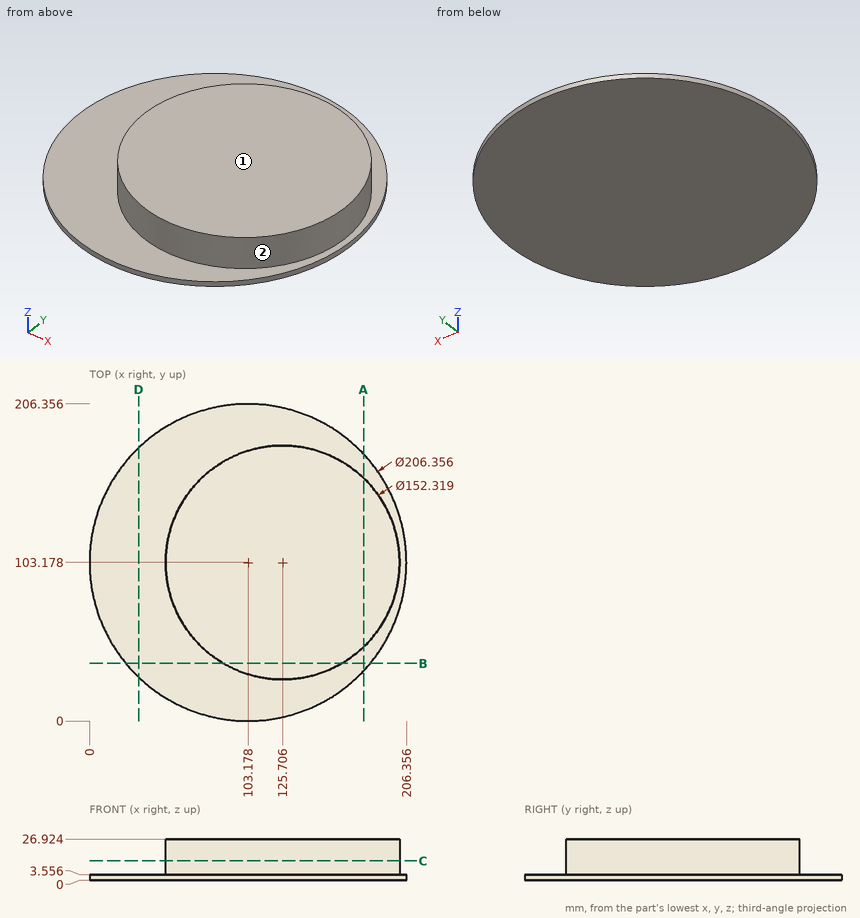
The drawing under review shows one solid part. Ordinate dimensions are in mm from its lowest x, y, z. A direction names the side the tool comes from. Give positions to 0.01 mm unless a question says otherwise; leave off trailing zeros. Loops run counter-clockwise (first coordinate to the right, second up) from the corner with the lowest first, then second, coordinate; pieces in that order, holes last. Notation, with made-up numbers: M -15.75,-13 L 43.25,-13 A21 cw 43.25,18 Z; hole C 32,87.5 d1. An arc over 180 degrees is marked long. Return JSON: item names as keys, results as strings. Group by question number.
Item 1: Tool access review of the marked faces 1 and 2: name each direction out of +Z, -Z, +X, -X, +Y, -Y from which nothing blocks a thin tool from reaching the whole face with its end or side.
Item 2: We need section C-C (z = 12.75). Give the boundary of the cut face in (x, y), and give its area (3 significant figures).
Item 3: For probe 1 along Z at (x, y) = (128, 22); probe 2 along X at (y, z) = (153.5, 7.25) (1 decimal); probe 3 along Y at (x, z) = (37, 3.5) (1 decimal), list the stretches that pass through material, from the lowest coordinate up.
Item 4: We need section D-D (x = 32). Give the boundary of the cut face in (y, z).
Item 5: We need section A-A (x = 178.5). Give the boundary of the cut face in (y, z) (1 decimal), and give its area (3 significant figures).
Item 6: We need section B-B (y = 37.5). Give the boundary of the cut face in (x, z) (1 decimal), and give its area (3 significant figures).
Item 7: Insertion check: pin 1 Ø2 at (y, z) = (95.5, 6) entering from -X; pin 2 Ø8 at (y, z) = (42.5, 20) entering from -X (1 decimal); pin 3 Ø5 at (x, z) = (167.5, 24) entering from -Y. Each pin has a flat end and moves straight along its axis. Give the tip position at first contact, or say it passes through.
Output:
{
 "1": {"face 1": "+Z, +X, -X, +Y, -Y", "face 2": "+Z"},
 "2": {"outline": "C 125.71,103.18 d152.32", "area": "18,200 mm^2"},
 "3": {"probe 1": "z = 0 to 3.56", "probe 2": "x = 68.5 to 182.9", "probe 3": "y = 24 to 182.3"},
 "4": {"outline": "M 28.48,0 L 177.87,0 L 177.87,3.56 L 28.48,3.56 Z"},
 "5": {"outline": "M 32.7,0 L 173.7,0 L 173.7,3.6 L 158.1,3.6 L 158.1,26.9 L 48.3,26.9 L 48.3,3.6 L 32.7,3.6 Z", "area": "3,070 mm^2"},
 "6": {"outline": "M 23.6,0 L 182.8,0 L 182.8,3.6 L 164.3,3.6 L 164.3,26.9 L 87.1,26.9 L 87.1,3.6 L 23.6,3.6 Z", "area": "2,370 mm^2"},
 "7": {"pin 1": "stops at x = 49.84", "pin 2": "stops at x = 74.8", "pin 3": "stops at y = 37.94"}
}
